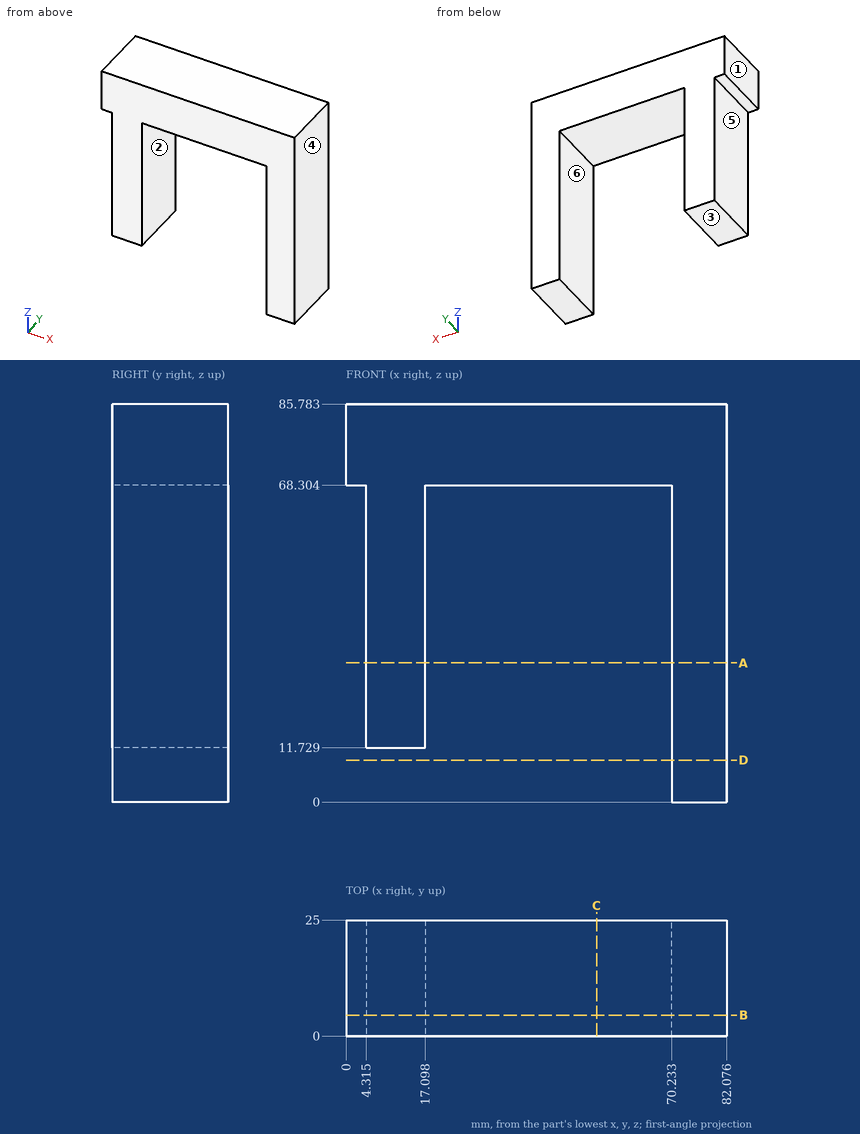
Source: three-view drawing plus pictorial views. Frame: mm from the lowest corner of the part. A direction names the side the tool comes from. Coordinates: 2 decimals unless noted, no trailing zeros. Loops run counter-clockwise (first coordinate to the right, second up) from the corner with the lowest first, then second, coordinate; pieces in that order, holes last. Notation, with made-up numbers: (15.5, 53.25) -> (49.5, 53.25) arc R25 cw to (49.5, 65.25) -> close; hole circle Ø1 at (55.25, 12). An arc over 180 degrees is marked (long way). One line per item, written item: value.
(1) Cut plane B-B (y = 4.5). Output: boundary loops of the cut face in (x, z) (1 decimal), then the cut area to 3 significant figures.
Answer below:
outline: (0, 68.3) -> (4.3, 68.3) -> (4.3, 11.7) -> (17.1, 11.7) -> (17.1, 68.3) -> (70.2, 68.3) -> (70.2, 0) -> (82.1, 0) -> (82.1, 85.8) -> (0, 85.8) -> close
area: 2,970 mm2
(2) Draft query along X for the marked faces 1, 2 and 3. Return one class per face: pulls with the +X half, pulls with the -X half, needs draft (parallel to the pull), parting line crosses it, or undercut.
Answer below:
face 1: pulls with the -X half
face 2: undercut
face 3: needs draft
(3) Cut plane D-D (z = 9). Output: boundary loops of the cut face in (x, y).
Answer below:
outline: (70.23, 0) -> (82.08, 0) -> (82.08, 25) -> (70.23, 25) -> close
(4) Cut plane C-C (x = 54). Output: boundary loops of the cut face in (y, z).
Answer below:
outline: (0, 68.3) -> (25, 68.3) -> (25, 85.78) -> (0, 85.78) -> close
(5) Set-up query: the marked faces 4, 5 and 6. Return all of +Z, -Z, +X, -X, +Y, -Y with unobstructed straight access to the full face (end or side cutting, diameter ignored); none if empty.
Answer below:
face 4: +Z, -Z, +X, +Y, -Y
face 5: -Z, -X, +Y, -Y
face 6: -Z, +Y, -Y
(6) Ray query, line 1 along X through (y, z) = (22, 14.5) (1 decimal); line 2 along Z through (x, y) = (69.5, 8.75); line 3 along Z through (x, y) = (15, 2.75). Return the intervals inside material, ascending.
Answer below:
line 1: x = 4.3 to 17.1, 70.2 to 82.1
line 2: z = 68.3 to 85.78
line 3: z = 11.73 to 85.78
(7) Pin query (flat end, axial travel): pin 1 Ø8 at (y, z) = (13, 51) entering from -X (1 decimal); pin 2 Ø7.5 at (x, y) = (31.5, 8.5) entering from -Z; pin 3 Ø4 at (x, y) = (11, 17.5) entering from -Z. Return the tip coordinate at first contact, or that it passes through.
Answer below:
pin 1: stops at x = 4.3
pin 2: stops at z = 68.3
pin 3: stops at z = 11.73
(8) Cut plane A-A (z = 30). Output: boundary loops of the cut face in (x, y) (1 decimal), then the cut area to 3 significant figures.
Answer below:
outline: (4.3, 0) -> (17.1, 0) -> (17.1, 25) -> (4.3, 25) -> close; (70.2, 0) -> (82.1, 0) -> (82.1, 25) -> (70.2, 25) -> close
area: 616 mm2
